from build123d import *

# Parameters (mm, degrees)
SKETCH1_W           = 550
SKETCH1_H           = 300
BOSS_EXTRUDE1_DEPTH = 6
FILLET1_R           = 3
SKETCH3_W           = 500
SKETCH3_H           = 250
BOSS_EXTRUDE2_DEPTH = 26
FILLET2_R           = 6


with BuildPart() as part:
    # Sketch1 → Boss-Extrude1 (new body)
    with BuildSketch(Plane(origin=(0, 0, 0), x_dir=(1, 0, 0), z_dir=(0, 1, 0))):
        with Locations((275, 150)):
            Rectangle(SKETCH1_W, SKETCH1_H)
    extrude(amount=BOSS_EXTRUDE1_DEPTH)

    # Fillet1
    fillet1_edges = [part.edges().sort_by_distance(p)[0] for p in [
        (550, 6, -150),
        (275, 6, -300),
        (0, 6, -150),
        (275, 6, 0),
    ]]
    fillet(fillet1_edges, radius=FILLET1_R)

    # Sketch3 → Boss-Extrude2 (add)
    with BuildSketch(Plane.XZ):
        with Locations((275, -150)):
            Rectangle(SKETCH3_W, SKETCH3_H)
    extrude(amount=BOSS_EXTRUDE2_DEPTH)

    # Fillet2
    fillet2_edges = [part.edges().sort_by_distance(p)[0] for p in [
        (25, -13, -275),
        (525, -13, -275),
        (525, -13, -25),
        (25, -13, -25),
        (275, -26, -275),
        (525, -26, -150),
        (275, -26, -25),
        (25, -26, -150),
    ]]
    fillet(fillet2_edges, radius=FILLET2_R)


solid = part.part
Here's how the part is built. I have some questions about the finished solid (model axes, mm). A direction names the side the tool comes from. Coordinates: 2 decimals unless noted, no trailing zeros. Write each loop counter-clockwise with the first axis right and the second up, starting at its lowest first coordinate (ties: lowest second). Pieces come first, ordered by that corner, then holes.
Item 1: Will these pins go through, and if not, where does the flat tip stop? pin 1 (2 mm diameter, centred on x = 434.5, y = -6, fed in from -Z); pin 2 (6 mm diameter, centred on y = -12, z = -126.5, fed in from -X); pin 3 (16 mm diameter, centred on x = 373.5, y = -14, fed in from +Z).
Item 2: I want a section at C-C on x = 203.5. Write out the boundary of the cut face in (y, z).
Item 3: I want a section at B-B on y = -6.5. Write out the boundary of the cut face in (x, z), and give its area (3 significant figures).
Item 4: On a 3-axis mill with a long thin cutter (end or side, diameter ignored), from which of +Z, -Z, +X, -X, +Y, -Y can I reach the whole of each face in a straight line? I mean faces 1 (the flat face through (525, -10, -152)), 2 (the flat face through (272, -10, -275)), 3 (the flat face through (253, 0, -17)). Say none if no direction works.
Item 5: If I drill on line 1 (X direction, y = 3.5, z = -123); line 2 (Z direction, x = 415, y = -17.5); line 3 (X direction, y = -2, z = -62.5), over which ranges is the centre line in solid material (lowest first)?
Item 6: I want a section at A-A on z = -131. Write out the boundary of the cut face in (x, y), and give its area (3 significant figures).
Findings below:
1. pin 1: stops at z = -275
1. pin 2: stops at x = 25
1. pin 3: stops at z = -25
2. outline: (-26, -269) arc R6 ccw to (-20, -275) - (0, -275) - (0, -300) - (3, -300) arc R3 ccw to (6, -297) - (6, -3) arc R3 ccw to (3, 0) - (0, 0) - (0, -25) - (-20, -25) arc R6 ccw to (-26, -31) - close
3. outline: (25, -269) arc R6 ccw to (31, -275) - (519, -275) arc R6 ccw to (525, -269) - (525, -31) arc R6 ccw to (519, -25) - (31, -25) arc R6 ccw to (25, -31) - close
3. area: 125,000 mm2
4. face 1: +Z, -Z, +X, -Y
4. face 2: -Z, +X, -X, -Y
4. face 3: -Y
5. line 1: x = 0.04 to 549.96
5. line 2: z = -275 to -25
5. line 3: x = 25 to 525
6. outline: (0, 0) - (25, 0) - (25, -20) arc R6 ccw to (31, -26) - (519, -26) arc R6 ccw to (525, -20) - (525, 0) - (550, 0) - (550, 3) arc R3 ccw to (547, 6) - (3, 6) arc R3 ccw to (0, 3) - close
6. area: 16,300 mm2
